Read the model definition and answer for the solid it produces. Units are mm, in the model's axes. Face numbers are marked on the shaded views. Coordinates: 2 decimals unless noted, no trailing zeros. Write each loop counter-clockwise with the first axis right and the second up, starting at its lowest first coordinate (ties: lowest second). Pieces come first, ordered by that corner, then holes. Notation, with made-up numbers: (57.5, 11) -> (72.5, 11) arc R17 ccw to (72.5, 30) -> close; hole circle Ø8 at (23, 85.25). An arc over 180 degrees is marked (long way). Return JSON: item names as keys, results as strings.
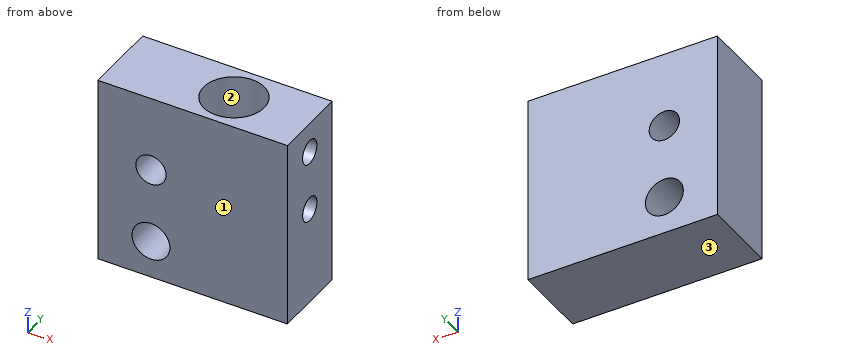
from build123d import *

# Parameters (mm, degrees)
F0_W     = 25
F0_H     = 25
F1_DEPTH = 5
F3_D     = 4
F4_D     = 5
F6_D     = 8
F6_DEPTH = 16
F6_TIP   = 2.4034424761
F8_D     = 3.2
F8_DEPTH = 10
F8_TIP   = 0.9613769904


with BuildPart() as f1:
    # F0 (on Front) → F1 (new body, symmetric)
    with BuildSketch(Plane.XZ):
        Rectangle(F0_W, F0_H)
    extrude(amount=F1_DEPTH, both=True)

    # F3 (through all)
    with Locations(Plane.XZ.offset(5)):
        with Locations((-5.5, 2.5)):
            Hole(F3_D / 2)

    # F4 (through all)
    with Locations(Plane.XZ.offset(5)):
        with Locations((-5.5, -7.5)):
            Hole(F4_D / 2)

    # F6
    with Locations(Plane.XY.offset(12.5)):
        with Locations((2.5, 0)):
            Hole(F6_D / 2, depth=F6_DEPTH)
            with Locations((0, 0, -(F6_DEPTH + F6_TIP / 2))):  # 118° drill point
                Cone(0, F6_D / 2, F6_TIP, mode=Mode.SUBTRACT)

    # F8
    with Locations(Plane.YZ.offset(12.5)):
        with Locations((0, 8.5), (0, 0.5)):
            Hole(F8_D / 2, depth=F8_DEPTH)
            with Locations((0, 0, -(F8_DEPTH + F8_TIP / 2))):  # 118° drill point
                Cone(0, F8_D / 2, F8_TIP, mode=Mode.SUBTRACT)


solid = f1.part
1. The part is cut by section D-D (x = 10.5). Determine the outline of the cut face in (y, z).
Taken from the geometry:
{"outline": "(-5, -12.5) -> (5, -12.5) -> (5, 12.5) -> (-5, 12.5) -> close; hole circle Ø3.2 at (0, 0.5); hole circle Ø3.2 at (0, 8.5)"}
2. The part is cut by section B-B (x = -5.5). Determine the outline of the cut face in (y, z), then the cut area to 3 significant figures.
Taken from the geometry:
{"outline": "(-5, -12.5) -> (5, -12.5) -> (5, -10) -> (-5, -10) -> close; (-5, -5) -> (5, -5) -> (5, 0.5) -> (-5, 0.5) -> close; (-5, 4.5) -> (5, 4.5) -> (5, 12.5) -> (-5, 12.5) -> close", "area": "160 mm2"}
3. For a pull along Y with two mould halves and no side action, classify the marked faces 1, 2 and 3 as +Y half, -Y half, draft (parallel to the pull), parting line (faces both ways), or undercut.
Taken from the geometry:
{"face 1": "-Y half", "face 2": "undercut", "face 3": "draft"}
4. The part is cut by section C-C (z = -7.5). Determine the outline of the cut face in (x, y).
Taken from the geometry:
{"outline": "(-12.5, -5) -> (-8, -5) -> (-8, 5) -> (-12.5, 5) -> close; (-3, -5) -> (12.5, -5) -> (12.5, 5) -> (-3, 5) -> close"}
5. Consider L1, parallel to Z at x = -5.5, y = 0.5; L2, parallel to Y at x = 9.5, z = 8.5; L3, parallel to Z at x = 8.5, y = 0. Determine where each line is inside the solid, lowest interval first.
Taken from the geometry:
{"L1": "z = -12.5 to -10, -5 to 0.5, 4.5 to 12.5", "L2": "y = -5 to -1.6, 1.6 to 5", "L3": "z = -12.5 to -1.1, 2.1 to 6.9, 10.1 to 12.5"}
6. The part is cut by section A-A (z = 2.5). Determine the outline of the cut face in (x, y).
Taken from the geometry:
{"outline": "(-12.5, -5) -> (-7.5, -5) -> (-7.5, 5) -> (-12.5, 5) -> close; (-3.5, -5) -> (12.5, -5) -> (12.5, 5) -> (-3.5, 5) -> close; hole circle Ø8 at (2.5, 0)"}
